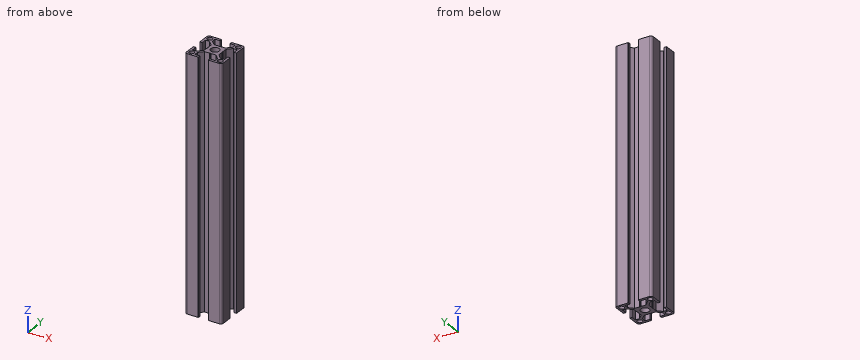
```python
from build123d import *

# Parameters (mm, degrees)
SKETCH1_R           = 2.1
SKETCH1_R_2         = 3.4
BOSS_EXTRUDE1_DEPTH = 204


with BuildPart() as part:
    # Sketch1 → Boss-Extrude1 (new body)
    with BuildSketch(Plane.XY):
        with BuildLine():
            Line((-14.7, 4), (-13, 4))
            Line((-13, 4), (-13, 8.25))
            Line((-13, 8.25), (-9.664213562, 8.25))
            Line((-9.664213562, 8.25), (-6, 4.585786438))
            Line((-6, 4.585786438), (-6, 0.519615242))
            Line((-6, 0.519615242), (-5.7, 0))
            Line((-5.7, 0), (-6, -0.519615242))
            Line((-6, -0.519615242), (-6, -4.585786438))
            Line((-6, -4.585786438), (-9.664213562, -8.25))
            Line((-9.664213562, -8.25), (-13, -8.25))
            Line((-13, -8.25), (-13, -4))
            Line((-13, -4), (-14.7, -4))
            ThreePointArc((-14.7, -4), (-14.912132034, -4.087867966), (-15, -4.3))
            Line((-15, -4.3), (-15, -13))
            ThreePointArc((-15, -13), (-14.414213562, -14.414213562), (-13, -15))
            Line((-13, -15), (-4.3, -15))
            ThreePointArc((-4.3, -15), (-4.087867966, -14.912132034), (-4, -14.7))
            Line((-4, -14.7), (-4, -13))
            Line((-4, -13), (-8.25, -13))
            Line((-8.25, -13), (-8.25, -9.664213562))
            Line((-8.25, -9.664213562), (-4.585786438, -6))
            Line((-4.585786438, -6), (-0.519615242, -6))
            Line((-0.519615242, -6), (0, -5.7))
            Line((0, -5.7), (0.519615242, -6))
            Line((0.519615242, -6), (4.585786438, -6))
            Line((4.585786438, -6), (8.25, -9.664213562))
            Line((8.25, -9.664213562), (8.25, -13))
            Line((8.25, -13), (4, -13))
            Line((4, -13), (4, -14.7))
            ThreePointArc((4, -14.7), (4.087867966, -14.912132034), (4.3, -15))
            Line((4.3, -15), (13, -15))
            ThreePointArc((13, -15), (14.414213562, -14.414213562), (15, -13))
            Line((15, -13), (15, -4.3))
            ThreePointArc((15, -4.3), (14.912132034, -4.087867966), (14.7, -4))
            Line((14.7, -4), (13, -4))
            Line((13, -4), (13, -8.25))
            Line((13, -8.25), (9.664213562, -8.25))
            Line((9.664213562, -8.25), (6, -4.585786438))
            Line((6, -4.585786438), (6, -0.519615242))
            Line((6, -0.519615242), (5.7, 0))
            Line((5.7, 0), (6, 0.519615242))
            Line((6, 0.519615242), (6, 4.585786438))
            Line((6, 4.585786438), (9.664213562, 8.25))
            Line((9.664213562, 8.25), (13, 8.25))
            Line((13, 8.25), (13, 4))
            Line((13, 4), (14.7, 4))
            ThreePointArc((14.7, 4), (14.912132034, 4.087867966), (15, 4.3))
            Line((15, 4.3), (15, 13))
            ThreePointArc((15, 13), (14.414213562, 14.414213562), (13, 15))
            Line((13, 15), (4.3, 15))
            ThreePointArc((4.3, 15), (4.087867966, 14.912132034), (4, 14.7))
            Line((4, 14.7), (4, 13))
            Line((4, 13), (8.25, 13))
            Line((8.25, 13), (8.25, 9.664213562))
            Line((8.25, 9.664213562), (4.585786438, 6))
            Line((4.585786438, 6), (0.519615242, 6))
            Line((0.519615242, 6), (0, 5.7))
            Line((0, 5.7), (-0.519615242, 6))
            Line((-0.519615242, 6), (-4.585786438, 6))
            Line((-4.585786438, 6), (-8.25, 9.664213562))
            Line((-8.25, 9.664213562), (-8.25, 13))
            Line((-8.25, 13), (-4, 13))
            Line((-4, 13), (-4, 14.7))
            ThreePointArc((-4, 14.7), (-4.087867966, 14.912132034), (-4.3, 15))
            Line((-4.3, 15), (-13, 15))
            ThreePointArc((-13, 15), (-14.414213562, 14.414213562), (-15, 13))
            Line((-15, 13), (-15, 4.3))
            ThreePointArc((-15, 4.3), (-14.912132034, 4.087867966), (-14.7, 4))
        make_face()
        with Locations((11.625, 11.625)):
            Circle(SKETCH1_R, mode=Mode.SUBTRACT)
        with Locations((11.625, -11.625)):
            Circle(SKETCH1_R, mode=Mode.SUBTRACT)
        Circle(SKETCH1_R_2, mode=Mode.SUBTRACT)
        with Locations((-11.625, -11.625)):
            Circle(SKETCH1_R, mode=Mode.SUBTRACT)
        with Locations((-11.625, 11.625)):
            Circle(SKETCH1_R, mode=Mode.SUBTRACT)
    extrude(amount=BOSS_EXTRUDE1_DEPTH)


solid = part.part
```
The model under review builds one solid part; all positions refer to its coordinate system, in mm. Give positions to 0.01 mm unless a question says otherwise; leave off trailing zeros. Answer in a Markdown table with one row per item. Add a question column.
1. Insertion check: P1, Ø4.5, axis at x = -2, z = 62.5, coming from the -Y side; P2, Ø1.2, axis at x = -3, z = 93.5, coming from the +Y side; P3, Ø0.8, axis at y = 14, z = 116.5, coming from the +X side. Each pin has a flat end and moves straight along its axis. Give the tip position at first contact, or say it passes through.
2. We need section A-A on z = 100.5. State how many separate pieces and enclosed holes the cut face has, then the cut area to 3 significant figures.
3. Wall thickness on line 1 along X through (y, z) = (11.5, 14); line 2 along Y through (x, z) = (-10.5, 174); line 3 along Y through (x, z) = (-12.5, 67): over which ranges is each line inside the solid? List them lowest first. Write a range as [from, to].
Ans:
| question | item | result |
|---|---|---|
| 1 | P1 | stops at y = -15 |
| 1 | P2 | stops at y = 6 |
| 1 | P3 | stops at x = 14.91 |
| 2 | separate pieces | 1 |
| 2 | enclosed holes | 5 |
| 2 | area | 332 mm^2 |
| 3 | line 1 | x = [-15, -13.72], [-9.53, -8.25], [8.25, 9.53], [13.72, 15] |
| 3 | line 2 | y = [-15, -13.4], [-9.85, -8.25], [8.25, 9.85], [13.4, 15] |
| 3 | line 3 | y = [-15, -13.53], [-9.72, -8.25], [8.25, 9.72], [13.53, 15] |
